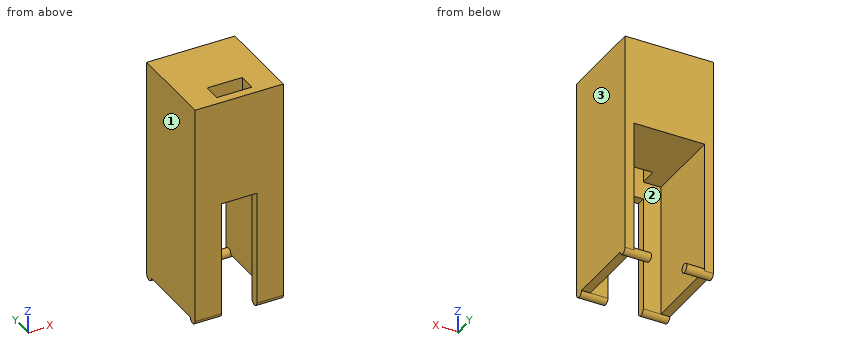
from build123d import *

# Parameters (mm, degrees)
SKETCH_1_W          = 20
SKETCH_1_H          = 50
EXTRUDE_1_DEPTH     = 20
SKETCH_2_W          = 16
SKETCH_2_H          = 30
CUT_EXTRUDE_1_DEPTH = 18
SKETCH_3_W          = 8
SKETCH_3_H          = 38.402735184
CUT_EXTRUDE_2_DEPTH = 18
SKETCH_4_R          = 1
EXTRUDE_2_DEPTH     = 6
SKETCH_5_R          = 1
EXTRUDE_3_DEPTH     = 6
SKETCH_6_W          = 8
SKETCH_6_H          = 4
CUT_EXTRUDE_3_DEPTH = 30


with BuildPart() as part:
    # 草图1 → 凸台-拉伸1 (new body)
    with BuildSketch(Plane(origin=(0, 0, 0), x_dir=(1, 0, 0), z_dir=(0, 1, 0))):
        with Locations((0, 5)):
            Rectangle(SKETCH_1_W, SKETCH_1_H)
    extrude(amount=EXTRUDE_1_DEPTH)

    # 草图2 → 切除-拉伸1 (cut)
    with BuildSketch(Plane(origin=(0, 20, 0), x_dir=(1, 0, 0), z_dir=(0, 1, 0))):
        with Locations((0, 15)):
            Rectangle(SKETCH_2_W, SKETCH_2_H)
    extrude(amount=-CUT_EXTRUDE_1_DEPTH, mode=Mode.SUBTRACT)

    # 草图3 → 切除-拉伸2 (cut)
    with BuildSketch(Plane.XZ):
        with Locations((0, -23.201367592)):
            Rectangle(SKETCH_3_W, SKETCH_3_H)
    extrude(amount=-CUT_EXTRUDE_2_DEPTH, mode=Mode.SUBTRACT)

    # 草图4 → 凸台-拉伸2 (add)
    with BuildSketch(Plane(origin=(-4, 0, 0), x_dir=(0, 0, -1), z_dir=(1, 0, 0))):
        with Locations((30, 1)):
            Circle(SKETCH_4_R)
        with Locations((30, 19)):
            Circle(SKETCH_4_R)
    extrude(amount=-EXTRUDE_2_DEPTH)

    # 草图5 → 凸台-拉伸3 (add)
    with BuildSketch(Plane.ZY.offset(-4)):
        with Locations((-30, 1)):
            Circle(SKETCH_5_R)
        with Locations((-30, 19)):
            Circle(SKETCH_5_R)
    extrude(amount=-EXTRUDE_3_DEPTH)

    # 草图6 → 切除-拉伸3 (cut)
    with BuildSketch(Plane(origin=(0, 0, 0), x_dir=(-1, 0, 0), z_dir=(0, 0, -1))):
        with Locations((0, 4)):
            Rectangle(SKETCH_6_W, SKETCH_6_H)
    extrude(amount=-CUT_EXTRUDE_3_DEPTH, mode=Mode.SUBTRACT)


solid = part.part
Read the model definition and answer for the solid it produces. Units are mm, in the model's axes. Face numbers are marked on the shaded views. Give positions to 0.01 mm unless a question says otherwise; leave off trailing zeros. Write each loop counter-clockwise with the first axis right and the second up, starting at its lowest first coordinate (ties: lowest second). Pieces come first, ordered by that corner, then holes. Notation, with made-up numbers: (69, 29) - (78, 29) arc R22 cw to (78, 46) - close; hole circle Ø8 at (59.5, 79). An arc over 180 degrees is marked (long way). Answer in a Markdown table with one row per item. Add a question column.
Item 1: Section D-D, the plane z = 16.5 is taken. Write down the section's boundary in (x, y).
Item 2: Section C-C, the plane y = 5.5 is taken. Write down the section's boundary in (x, z).
Item 3: Section A-A, the plane z = -23 is taken. Write down the section's boundary in (x, y), and give its area (3 significant figures).
Item 4: Determine the mould class of the marked faces 1, 2 and 3 for opening direction X: pulls with the +X half, pulls with the -X half, needs draft (parallel to the pull), parting line crosses it, or undercut.
Item 5: Flat-ended cylindrical pins translate along their axes: P1, Ø6.5, axis at x = 0.5, z = 7, coming from the -Y side; P2, Ø1.5, axis at x = -6, y = 7, coming from the -Z side; P3, Ø1.6, axis at x = 1.5, y = 1, coming from the -Z side; P4, Ø2, axis at x = 9.5, y = 12, coming from the -Z side. Find the tip coordinate at first contact, or state that the pin passes through.
Item 6: Section B-B, the plane x = 7 is taken. Write down the section's boundary in (y, z).
Item 7: Find the intervals of material crossed by L1, parallel to X at y = 18.75, z = -17; L2, parallel to X at y = 5, z = 4.5; L3, parallel to Y at x = 3, z = 1.5, in increasing order.
Recorded:
| question | item | result |
|---|---|---|
| 1 | outline | (-10, 0) - (10, 0) - (10, 20) - (-10, 20) - close; hole (-4, 2) - (4, 2) - (4, 6) - (-4, 6) - close |
| 2 | outline | (-10, -30) - (-8, -30) - (-8, 0) - (-4, 0) - (-4, 20) - (-10, 20) - close; (4, 0) - (8, 0) - (8, -30) - (10, -30) - (10, 20) - (4, 20) - close |
| 3 | outline | (-10, 0) - (-4, 0) - (-4, 2) - (-8, 2) - (-8, 20) - (-10, 20) - close; (4, 0) - (10, 0) - (10, 20) - (8, 20) - (8, 2) - (4, 2) - close |
| 3 | area | 96.0 mm2 |
| 4 | face 1 | pulls with the -X half |
| 4 | face 2 | undercut |
| 4 | face 3 | pulls with the +X half |
| 5 | P1 | stops at y = 0 |
| 5 | P2 | stops at z = 0 |
| 5 | P3 | stops at z = -4 |
| 5 | P4 | stops at z = -30 |
| 6 | outline | (0, -30) arc R1 ccw to (2, -30) - (2, 0) - (20, 0) - (20, 20) - (0, 20) - close; circle Ø2 at (19, -30) |
| 7 | L1 | x = -10 to -8, 8 to 10 |
| 7 | L2 | x = -10 to -4, 4 to 10 |
| 7 | L3 | y = 0 to 2, 6 to 20 |
